Build history of the part. All positions in model axes, mm. Face numbers are marked on the shaded views. A direction names the side the tool comes from. Give positions to 0.01 mm unless a question says otherwise; leave off trailing zeros. Order: outer loops, then holes, each group sorted by start corner. A loop starts at its lowest first (then second) coordinate and runs counter-clockwise, first axis right, second up. Notation, with made-up numbers: (-1, 42.5) -> (26, 42.5) arc R35 cw to (26, 78.5) -> close; hole circle Ø11 at (-27.5, 43). An arc over 180 degrees is marked (long way). One line per item, written item: value. Start each with the question number.
(1) Saw through at B-B on y = -1. Give the cut face in (x, z), plus the area to 3 significant figures.
(2) Saw through at A-A on x = -3. Give the cut face in (y, z), plus the area to 3 significant figures.
(3) Pin check, flat tips, straight feed: pin 1 (1.5 mm diameter, centred on y = 9.5, z = 3.5, fed in from -X); pin 2 (2.5 mm diameter, centred on y = 11.5, z = 2.5, fed in from +X); pin 3 (3 mm diameter, centred on x = 20, z = 3, fed in from -Y); pin 4 (1.5 mm diameter, centred on x = 2, z = 1.5, fed in from -Y). Stop position of each tip, or through.
(4) Saw through at C-C on x = 12.5. Give the cut face in (y, z), plus the area to 4 significant figures.
(5) Which spindle directions (+Z, -Z, +X, -X, +Y, -Y) get a long thin tool onto all of the face, cutting with end or side? Do the marked faces 4 and 5. Say none if no direction does.
(6) Two-plate mould, pull along X, no slides. Class the marked faces 1, 2 and 3: +X half, -X half, draft (parallel to the pull), parting line (faces both ways), or undercut.
(7) Probe line 1 (X direction, y = 6, z = 3.4); line 2 (Y direction, x = -4, z = 4.4); line 3 (X direction, y = 19.5, z = 1.8). List the from-to ranges inside material, lowest first.
(8) Saw through at D-D on z = 2.65. Give the cut face in (x, y) (3 decimals).
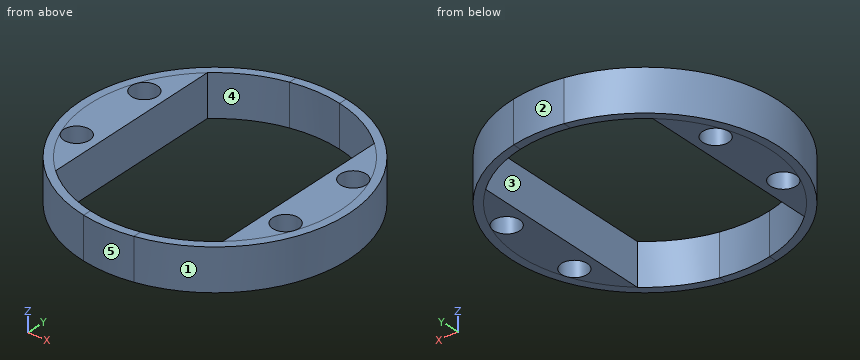
Autodesk Inventor part; units mm, degrees
ref_plane "YZ Plane" through (0, 0, 0) normal (1, 0, 0) x (0, 1, 0)
ref_plane "XZ Plane" through (0, 0, 0) normal (0, 1, 0) x (-1, 0, 0)
ref_plane "XY Plane" through (0, 0, 0) normal (0, 0, 1) x (1, 0, 0)
sketch "Sketch1" plane through (0, 0, 0) normal (0, 0, 1) x (1, 0, 0)
  line L0 (19.067, 0.7556) -> (19.067, 23.1833)
  arc A0 (19.067, 0.7556) -> (19.067, 23.1833) centre (9.067, 11.9694) ccw
  line L1 (-0.933, 23.1833) -> (-0.933, 0.7556)
  arc A1 (-0.933, 23.1833) -> (-0.933, 0.7556) centre (9.067, 11.9694) ccw
  line L2 (12.067, -2.753) -> (12.067, -3.7468)
  arc A2 (12.067, -3.7468) -> (12.067, 27.6857) centre (9.067, 11.9694) ccw
  line L3 (12.067, 27.6857) -> (12.067, 26.6919)
  arc A3 (12.067, -2.753) -> (12.067, 26.6919) centre (9.067, 11.9694) ccw
  line L4 (6.067, -3.7468) -> (6.067, -2.753)
  arc A4 (6.067, 26.6919) -> (6.067, -2.753) centre (9.067, 11.9694) ccw
  line L5 (6.067, 26.6919) -> (6.067, 27.6857)
  arc A5 (6.067, 27.6857) -> (6.067, -3.7468) centre (9.067, 11.9694) ccw
  arc A6 (12.067, 27.6857) -> (6.067, 27.6857) centre (9.067, 11.9694) ccw
  arc A7 (6.067, -3.7468) -> (12.067, -3.7468) centre (9.067, 11.9694) ccw
  circle A8 centre (9.067, 11.9694) radius 15.025
  point P0 (12.067, -2.753)
  point P1 (6.067, -2.753)
extrude "Extrusion1" add sketch "Sketch1" along normal blind 5 contours L0 A0 | A0 A3 L3 A2 L2 | L2 A7 L4 A8 | A8 L5 A6 L3 | L4 A5 L5 A4 A1 | A1 L1
sketch "Sketch2" plane through (9.067, 11.9694, 5) normal (0, 0, 1) x (1, 0, 0)
  circle A0 centre (12.5, 5) radius 1.55
  circle A1 centre (12.5, -5) radius 1.55
  circle A2 centre (-12.5, -5) radius 1.55
  circle A3 centre (-12.5, 5) radius 1.55
  circle A4 centre (0, 0) radius 16
  point P0 (-9.067, -11.9694)
extrude "Extrusion2" cut sketch "Sketch2" against normal through all contours A0 | A1 | A2 | A3
properties part number "arm_head_back"
Results below:
1. outline: (-0.3, 0) -> (1.48, 0) -> (1.48, 5) -> (-0.3, 5) -> close; (16.65, 0) -> (18.44, 0) -> (18.44, 5) -> (16.65, 5) -> close
1. area: 17.8 mm²
2. outline: (1.46, 0) -> (5.48, 0) -> (5.48, 5) -> (1.46, 5) -> close; (8.46, 0) -> (15.48, 0) -> (15.48, 5) -> (8.46, 5) -> close; (18.46, 0) -> (22.48, 0) -> (22.48, 5) -> (18.46, 5) -> close
2. area: 75.3 mm²
3. pin 1: stops at x = -6.84
3. pin 2: stops at x = 25.07
3. pin 3: stops at y = -0.95
3. pin 4: stops at y = -2.73
4. outline: (-3.66, 0) -> (-2.66, 0) -> (-2.66, 5) -> (-3.66, 5) -> close; (26.6, 0) -> (27.6, 0) -> (27.6, 5) -> (26.6, 5) -> close
4. area: 10.00 mm²
5. face 4: +Z, -Z
5. face 5: +Z, -Z, -Y
6. face 1: +X half
6. face 2: parting line
6. face 3: undercut
7. line 1: x = -5.78 to -4.64, -2.22 to -0.93, 19.07 to 20.36, 22.78 to 23.91
7. line 2: y = 2.74 to 5.53, 8.41 to 15.53, 18.41 to 21.2
7. line 3: x = -5.05 to -0.93, 19.07 to 23.18
8. outline: (6.067, -3.747) arc R16 ccw to (12.067, -3.747) arc R16 ccw to (12.067, 27.686) arc R16 ccw to (6.067, 27.686) arc R16 ccw to start; hole circle Ø3.1 at (-3.433, 6.969); hole circle Ø3.1 at (-3.433, 16.969); hole (-0.933, 0.756) arc R15.025 ccw to (6.067, -2.753) arc R15.025 ccw to (12.067, -2.753) arc R15.025 ccw to (19.067, 0.756) -> (19.067, 23.183) arc R15.025 ccw to (12.067, 26.692) arc R15.025 ccw to (6.067, 26.692) arc R15.025 ccw to (-0.933, 23.183) -> close; hole circle Ø3.1 at (21.567, 6.969); hole circle Ø3.1 at (21.567, 16.969)
